```python
from build123d import *

# Parameters (mm, degrees)
SKETCH5_W           = 146
SKETCH5_H           = 146
BOSS_EXTRUDE2_DEPTH = 250
FILLET8_R           = 40
FILLET9_R           = 40
FILLET10_R          = 40
FILLET11_R          = 40
FILLET12_R          = 10
BOSS_EXTRUDE5_START = -240
BOSS_EXTRUDE5_DEPTH = 240
SKETCH8_R           = 60
CUT_EXTRUDE1_DEPTH  = 34
SKETCH10_W          = 44
SKETCH10_H          = 33
CUT_EXTRUDE2_DEPTH  = 3
CUT_EXTRUDE3_DEPTH  = 3
SKETCH12_W          = 157.188162186
SKETCH12_H          = 158.114359626
CUT_EXTRUDE4_DEPTH  = 107
SKETCH15_W          = 32
SKETCH15_H          = 13
CUT_EXTRUDE7_DEPTH  = 5
CUT_EXTRUDE9_DEPTH  = 5


# Read off the part's stored shape, not the designer's step: Boss-Extrude5
with BuildPart() as part:
    # Sketch5 → Boss-Extrude2 (new body)
    with BuildSketch(Plane(origin=(0, 0, 0), x_dir=(1, 0, 0), z_dir=(0, 1, 0))):
        Rectangle(SKETCH5_W, SKETCH5_H)
    extrude(amount=BOSS_EXTRUDE2_DEPTH)

    # Fillet8
    fillet8_edges = [part.edges().sort_by_distance(p)[0] for p in [
        (73, 125, 73),
    ]]
    fillet(fillet8_edges, radius=FILLET8_R)

    # Fillet9
    fillet9_edges = [part.edges().sort_by_distance(p)[0] for p in [
        (73, 125, -73),
    ]]
    fillet(fillet9_edges, radius=FILLET9_R)

    # Fillet10
    fillet10_edges = [part.edges().sort_by_distance(p)[0] for p in [
        (-73, 125, -73),
    ]]
    fillet(fillet10_edges, radius=FILLET10_R)

    # Fillet11
    fillet11_edges = [part.edges().sort_by_distance(p)[0] for p in [
        (-73, 125, 73),
    ]]
    fillet(fillet11_edges, radius=FILLET11_R)

    # Fillet12
    fillet12_edges = [part.edges().sort_by_distance(p)[0] for p in [
        (73, 250, 0),
        (61.284271247, 250, 61.284271247),
        (0, 250, -73),
        (61.284271247, 250, -61.284271247),
        (-73, 250, 0),
        (-61.284271247, 250, -61.284271247),
        (0, 250, 73),
        (-61.284271247, 250, 61.284271247),
    ]]
    fillet(fillet12_edges, radius=FILLET12_R)

    # Boss-Extrude5 outline → Boss-Extrude5 (cut)
    with BuildSketch(Plane.XZ.offset(BOSS_EXTRUDE5_START)):
        with BuildLine():
            Line((30, 70), (-30, 70))
            ThreePointArc((-30, 70), (-58.284271247, 58.284271247), (-70, 30))
            Line((-70, 30), (-70, -30))
            ThreePointArc((-70, -30), (-58.284271247, -58.284271247), (-30, -70))
            Line((-30, -70), (30, -70))
            ThreePointArc((30, -70), (58.284271247, -58.284271247), (70, -30))
            Line((70, -30), (70, 30))
            ThreePointArc((70, 30), (58.284271247, 58.284271247), (30, 70))
        make_face()
    extrude(amount=BOSS_EXTRUDE5_DEPTH, mode=Mode.SUBTRACT)

    # Sketch8 → Cut-Extrude1 (cut)
    with BuildSketch(Plane(origin=(0, 250, 0), x_dir=(1, 0, 0), z_dir=(0, 1, 0))):
        with Locations(Location((0, 0, 0), (0, 0, 270))):
            Circle(SKETCH8_R)
    extrude(amount=-CUT_EXTRUDE1_DEPTH, mode=Mode.SUBTRACT)

    # Sketch10 → Cut-Extrude2 (cut)
    with BuildSketch(Plane(origin=(73, 0, 0), x_dir=(0, 0, -1), z_dir=(1, 0, 0))):
        with Locations((0, 63.5)):
            Rectangle(SKETCH10_W, SKETCH10_H)
    extrude(amount=-CUT_EXTRUDE2_DEPTH, mode=Mode.SUBTRACT)

    # Sketch11 → Cut-Extrude3 (cut)
    with BuildSketch(Plane.ZY.offset(73)):
        Polygon((0, 0), (-16, 0), (-16, 13), (16, 13), (16, 0), align=None)
    extrude(amount=-CUT_EXTRUDE3_DEPTH, mode=Mode.SUBTRACT)

    # Sketch12 → Cut-Extrude4 (cut)
    with BuildSketch(Plane.XZ):
        with Locations((-1.675039252, -2.437620076)):
            Rectangle(SKETCH12_W, SKETCH12_H)
    extrude(amount=-CUT_EXTRUDE4_DEPTH, mode=Mode.SUBTRACT)

    # Sketch15 → Cut-Extrude7 (cut)
    with BuildSketch(Plane.ZY.offset(73)):
        with Locations((0, 113.5)):
            Rectangle(SKETCH15_W, SKETCH15_H)
    extrude(amount=-CUT_EXTRUDE7_DEPTH, mode=Mode.SUBTRACT)

    # Sketch17 → Cut-Extrude9 (cut)
    with BuildSketch(Plane.ZY.offset(-70)):
        with BuildLine():
            Line((30, 154), (-30, 154))
            Line((-30, 154), (-30, 198.899888641))
            ThreePointArc((-30, 198.899888641), (0, 208), (30, 198.899888641))
            Line((30, 198.899888641), (30, 154))
        make_face()
    extrude(amount=-CUT_EXTRUDE9_DEPTH, mode=Mode.SUBTRACT)


solid = part.part
```
Geometry: final body of the model. Coordinates: model frame, mm. A direction names the side the tool comes from. Round coordinates to 2 decimals unless told otherwise and drop trailing zeros. Order: outer loops, then holes, each group sorted by start corner. A loop starts at its lowest first (then second) coordinate and runs counter-clockwise, first axis right, second up. Notation, with made-up numbers: M 19,72.25 L 39,72.25 A21 ccw 39,90.25 Z; hole C 19.5,8.25 d4. An arc over 180 degrees is marked long. One line per item, written item: value.
(1) Pin query (flat end, axial travel): P1, Ø3.5, axis at x = -71.5, z = -7, coming from the -Y side; P2, Ø0.9, axis at x = 72, z = 14.5, coming from the +Y side; P3, Ø2.5, axis at x = 71, y = 184, coming from the -Z side. Return the tip coordinate at first contact, or that it passes through.
Result sheet:
P1: y = 120
P2: y = 245.19
P3: z = -48.79
(2) Cut plane B-B (x = 0). Return the cut outline in (y, z), and give its area (3 significant figures).
Result sheet:
outline: M 107,-73 L 240,-73 A10 ccw 250,-63 L 250,-60 L 240,-60 L 240,-70 L 107,-70 Z; M 107,70 L 240,70 L 240,60 L 250,60 L 250,63 A10 ccw 240,73 L 107,73 Z
area: 1,020 mm2
(3) Pull-direction query (Z, two-part tool) for faces 4 (the cylindrical face through (60.972, 174.431, 61.594)), 5 (the flat face through (-11, 107, 71)), 6 (the flat face through (-63, 240, 1)); classes: pulls with the +Z half, pulls with the -Z half, needs draft (parallel to the pull), parting line crosses it, or undercut.
Result sheet:
face 4: pulls with the +Z half
face 5: needs draft
face 6: undercut
(4) Cut plane D-D (y = 191). Return the cut outline in (x, z).
Result sheet:
outline: M -73,-33 A40 ccw -33,-73 L 33,-73 A40 ccw 73,-33 L 73,-30 L 70,-30 A40 cw 30,-70 L -30,-70 A40 cw -70,-30 L -70,30 A40 cw -30,70 L 30,70 A40 cw 70,30 L 73,30 L 73,33 A40 ccw 33,73 L -33,73 A40 ccw -73,33 Z
(5) Cut plane A-A (z = 0). Return the cut outline in (x, y), and give its area (3 significant figures).
Result sheet:
outline: M -73,120 L -70,120 L -70,240 L -60,240 L -60,250 L -63,250 A10 ccw -73,240 Z; M 60,240 L 70,240 L 70,208 L 73,208 L 73,240 A10 ccw 63,250 L 60,250 Z; M 70,107 L 73,107 L 73,154 L 70,154 Z
area: 814 mm2
(6) Reachability of faces 1 (the cylindrical face through (58.594, 174.431, 57.972)), 2 (the cylindrical face through (0.46, 246.99, 70.15)), 3 (the cylindrical face through (71, 208, 0)) from +Z, -Z, +X, -X, +Y, -Y: full face, straight path, thin tool, end or side. Return the list, or none.
Result sheet:
face 1: -Y
face 2: +Z, +X, -X, +Y
face 3: +X
(7) Line query: probe 1 along Z at (x, y) = (2, 115); probe 2 along X at (y, z) = (195, -6). Output: solid intervals per line, ascending. Write a range as [from, to].
Result sheet:
probe 1: [-73, -70], [70, 73]
probe 2: [-73, -70]
(8) Cut plane C-C (y = 132). Return the cut outline in (x, z), and give its area (3 significant figures).
Result sheet:
outline: M -73,-33 A40 ccw -33,-73 L 33,-73 A40 ccw 73,-33 L 73,33 A40 ccw 33,73 L -33,73 A40 ccw -73,33 Z; hole M -70,-30 A40 ccw -30,-70 L 30,-70 A40 ccw 70,-30 L 70,30 A40 ccw 30,70 L -30,70 A40 ccw -70,30 Z
area: 1,720 mm2
